Print and shaded views of the part. All mm, measured from the part's lowest x, y and z. A direction names the side the tool comes from. Coordinates: 2 decimals unless noted, no trailing zeros. Loops run counter-clockwise (first coordinate to the right, second up) from the corner with the lowest first, then second, coordinate; pieces in that order, holes last. Notation, with made-up numbers: M 82.25,23.25 L 123.25,23.25 A18 ccw 123.25,52.25 Z; hole C -22,29 d2. An arc over 180 degrees is marked long. Use a Markdown table: item, result. Add a question column.
1) Tool access for the marked faces 1 and 2: list every direction of +Z, -Z, +X, -X, +Y, -Y with a clear straight run to the whole face (end or side of a thin tool).
2) Band-saw the part on A-A (z = 2.5). List the corners of the cut face in (x, y).
3) Pin check, flat tips, straight feed: pin 1 Ø2 at (x, z) = (8.5, 3.5) entering from +Y (1 decimal); pin 2 Ø1 at (y, z) = (2.5, 5.5) entering from +X. Stop position of each tip, or through.
4) Band-saw the part on B-B (y = 1.25). List the corners of the cut face in (x, z), plus the area to 3 significant figures.
5) Band-saw the part on C-C (x = 5.25). List the corners of the cut face in (y, z).
6) Wall check: probe 1 along X at (y, z) = (2.25, 4.75); probe 2 along Y at (x, z) = (4, 5.25); probe 3 along X at (y, z) = (4.75, 9.5). Give the ranges that are in metal, low to high. Write a range as from..to.
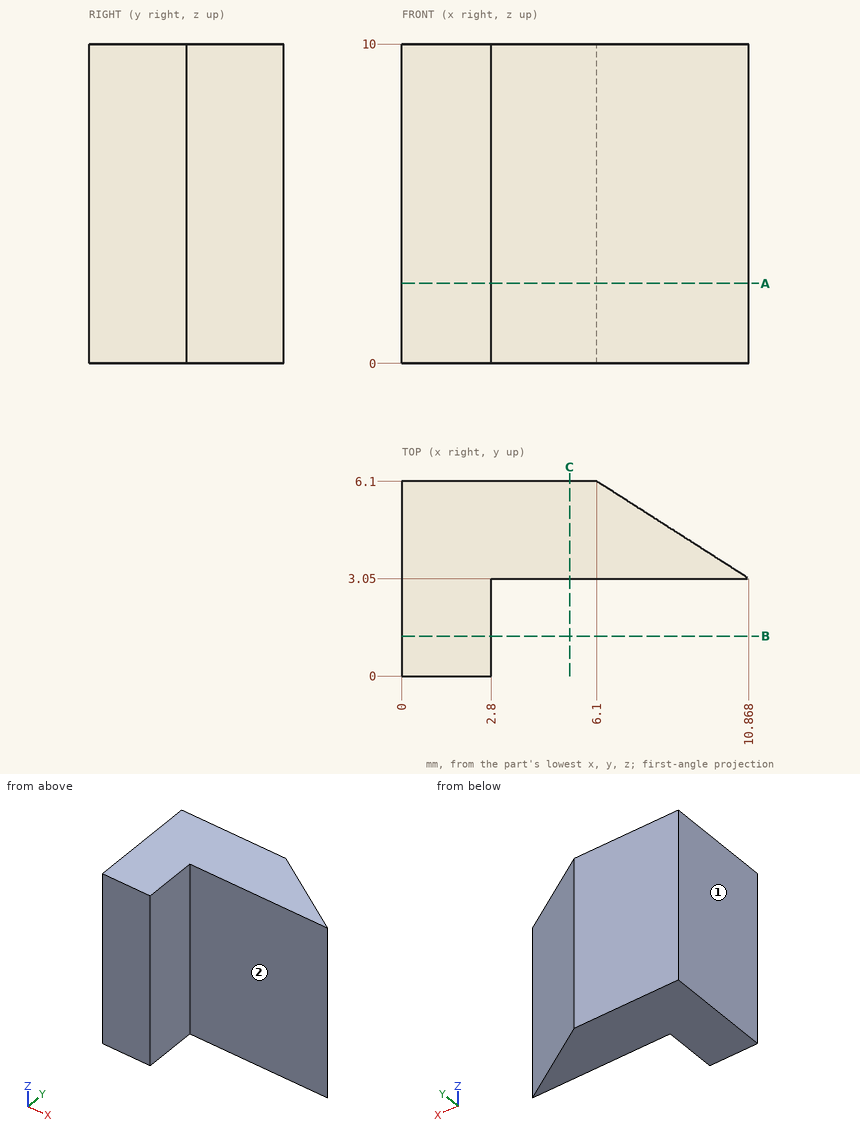
Entries:
| question | item | result |
|---|---|---|
| 1 | face 1 | +Z, -Z, -X, +Y, -Y |
| 1 | face 2 | +Z, -Z, +X, -Y |
| 2 | outline | M 0,0 L 2.8,0 L 2.8,3.05 L 10.87,3.05 L 6.1,6.1 L 0,6.1 Z |
| 3 | pin 1 | y = 5.2 |
| 3 | pin 2 | x = 2.8 |
| 4 | outline | M 0,0 L 2.8,0 L 2.8,10 L 0,10 Z |
| 4 | area | 28.0 mm2 |
| 5 | outline | M 3.05,0 L 6.1,0 L 6.1,10 L 3.05,10 Z |
| 6 | probe 1 | 0..2.8 |
| 6 | probe 2 | 3.05..6.1 |
| 6 | probe 3 | 0..8.21 |
